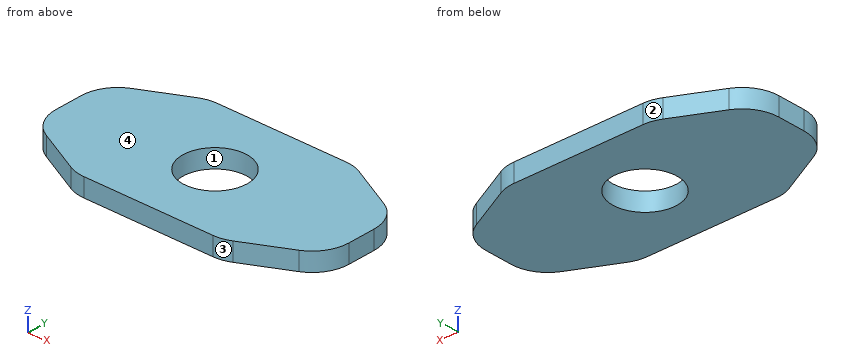
```python
from build123d import *

# Parameters (mm, degrees)
F0_R     = 5.55625
F1_DEPTH = 3.175
F2_R     = 6.35


with BuildPart() as f1:
    # F0 (on Top) → F1 (new body)
    with BuildSketch(Plane.XY):
        Polygon((-12.7, 12.7), (-25.4, 6.35), (-25.4, -6.35), (-12.7, -12.7), (12.7, -12.7), (25.4, -6.35), (25.4, 6.35), (12.7, 12.7), align=None)
        Circle(F0_R, mode=Mode.SUBTRACT)
    extrude(amount=F1_DEPTH)

    # F2
    f2_edges = [f1.edges().sort_by_distance(p)[0] for p in [
        (-12.7, -12.7, 1.5875),
        (12.7, -12.7, 1.5875),
        (25.4, -6.35, 1.5875),
        (25.4, 6.35, 1.5875),
        (12.7, 12.7, 1.5875),
        (-12.7, 12.7, 1.5875),
        (-25.4, 6.35, 1.5875),
        (-25.4, -6.35, 1.5875),
    ]]
    fillet(f2_edges, radius=F2_R)


solid = f1.part
```
Model file for the job. Use its own axes, mm. Face numbers are marked on the shaded views. Coordinates: 2 decimals unless noted, no trailing zeros. Loops run counter-clockwise (first coordinate to the right, second up) from the corner with the lowest first, then second, coordinate; pieces in that order, holes last. Notation, with made-up numbers: (-32.5, 65.5) - (-17.5, 65.5) arc R17 cw to (-17.5, 82.5) - close; hole circle Ø6 at (13, 60.25). An arc over 180 degrees is marked (long way). Answer as a JSON object with one key per item and string values. Group by question number.
(1) Cut at D-D (y = 10.5). Give the cut face in (x, z) (3 decimals).
(2) Two-plate mould, pull along Y, no slides. Class the marked faces 1, 2, 3 and 4: released by +Y, released by -Y, zero draft, split by the parting line, or undercut.
(3) Cut at B-B (y = 0). Give the cut face in (x, z) (3 decimals), then the cut area to 3 significant figures.
(4) Probe line 1 along Y through (x, z) = (0, 0.75); line 2 along Y through (x, z) = (5, 0.4); line 3 along X through (y, z) = (2.5, 1.4). List the from-to ranges inside material, lowest first.
(5) Flat gauge pins, fed straight in: pin 1 (8 mm diameter, centred on x = -12, y = 2, fed in from -Z); pin 2 (10 mm diameter, centred on x = 0, y = 0, fed in from -Z). Where does each tip first touch, or does it go through?
(6) Cut at A-A (x = 0). Give the cut face in (y, z) (3 decimals).
(7) Cut at C-C (z = 2.1). Give the cut face in (x, y), then the cut area to 3 significant figures.
Geometry says:
{
 "1": {"outline": "(-17.1, 0) - (17.1, 0) - (17.1, 3.175) - (-17.1, 3.175) - close"},
 "2": {"face 1": "undercut", "face 2": "released by +Y", "face 3": "released by -Y", "face 4": "zero draft"},
 "3": {"outline": "(-25.4, 0) - (-5.556, 0) - (-5.556, 3.175) - (-25.4, 3.175) - close; (5.556, 0) - (25.4, 0) - (25.4, 3.175) - (5.556, 3.175) - close", "area": "126 mm^2"},
 "4": {"line 1": "y = -12.7 to -5.56, 5.56 to 12.7", "line 2": "y = -12.7 to -2.42, 2.42 to 12.7", "line 3": "x = -25.4 to -4.96, 4.96 to 25.4"},
 "5": {"pin 1": "stops at z = 0", "pin 2": "passes through"},
 "6": {"outline": "(-12.7, 0) - (-5.556, 0) - (-5.556, 3.175) - (-12.7, 3.175) - close; (5.556, 0) - (12.7, 0) - (12.7, 3.175) - (5.556, 3.175) - close"},
 "7": {"outline": "(-25.4, -2.43) arc R6.35 ccw to (-21.89, -8.11) - (-14.04, -12.03) arc R6.35 ccw to (-11.2, -12.7) - (11.2, -12.7) arc R6.35 ccw to (14.04, -12.03) - (21.89, -8.11) arc R6.35 ccw to (25.4, -2.43) - (25.4, 2.43) arc R6.35 ccw to (21.89, 8.11) - (14.04, 12.03) arc R6.35 ccw to (11.2, 12.7) - (-11.2, 12.7) arc R6.35 ccw to (-14.04, 12.03) - (-21.89, 8.11) arc R6.35 ccw to (-25.4, 2.43) - close; hole circle Ø11.11 at (0, 0)", "area": "1,020 mm^2"}
}
